Design review of the part built by this model. Coordinates are the model's own, in mm. A direction names the side the tool comes from. Round coordinates to 2 decimals unless told otherwise and drop trailing zeros. Order: outer loops, then holes, each group sorted by start corner. A loop starts at its lowest first (then second) coordinate and runs counter-clockwise, first axis right, second up.
from build123d import *

# Parameters (mm, degrees)
SKETCH1_W           = 50
SKETCH1_H           = 20
BOSS_EXTRUDE1_DEPTH = 40
SKETCH2_W           = 45
SKETCH2_H           = 75.2
CUT_EXTRUDE1_DEPTH  = 15
CUT_EXTRUDE2_REACH  = 86.41
SKETCH3_W           = 8
SKETCH3_H           = 3
SKETCH4_W           = 30
SKETCH4_H           = 60
CUT_EXTRUDE3_DEPTH  = 1


with BuildPart() as part:
    # Sketch1 → Boss-Extrude1 (new, symmetric)
    with BuildSketch(Plane.XY):
        Rectangle(SKETCH1_W, SKETCH1_H)
    extrude(amount=BOSS_EXTRUDE1_DEPTH, both=True)

    # Sketch2 → Cut-Extrude1 (cut)
    with BuildSketch(Plane(origin=(0, 10, 0), x_dir=(1, 0, 0), z_dir=(0, 1, 0))):
        with Locations((0, -1.4)):
            Rectangle(SKETCH2_W, SKETCH2_H)
    extrude(amount=-CUT_EXTRUDE1_DEPTH, mode=Mode.SUBTRACT)

    # Sketch3 → Cut-Extrude2 (cut, up to next)
    with BuildSketch(Plane.XY.offset(40), mode=Mode.PRIVATE) as cut_extrude2_sk1:
        with Locations((0, -3.5)):
            Rectangle(SKETCH3_W, SKETCH3_H)
    cut_extrude2_tool1 = extrude(cut_extrude2_sk1.sketch, amount=-CUT_EXTRUDE2_REACH, mode=Mode.PRIVATE) & part.part
    add(cut_extrude2_tool1.solids().sort_by_distance((0, -3.5, 40))[0], mode=Mode.SUBTRACT)

    # Sketch4 → Cut-Extrude3 (cut)
    with BuildSketch(Plane(origin=(0, -5, 0), x_dir=(1, 0, 0), z_dir=(0, 1, 0))):
        with Locations((0, -9)):
            Rectangle(SKETCH4_W, SKETCH4_H)
    extrude(amount=-CUT_EXTRUDE3_DEPTH, mode=Mode.SUBTRACT)


solid = part.part
1) Clearance check with a flat-ended pin moving along its axis: P1, Ø5, axis at x = -18.5, z = -7.5, coming from the +Y side. State where the tip first meets the part, or that it passes through.
Results:
P1: stops at y = -5
2) For faces 5 (the face through (-25, 0, 1)), 6 (the face through (0, 3, -36.2)), list the 3-axis set-ups (+Z, -Z, +X, -X, +Y, -Y) from which the entire face can be reached by the end or side of a thin tool; tool diameter is ignored.
Results:
face 5: +Z, -Z, -X, +Y, -Y
face 6: +Y
3) The part is to be moulded in two halves that separate along Z. For faces 1 (the face through (0, 0, -40)), 2 (the face through (0, -10, 1)), 3 (the face through (0, 0, 40)), 4 (the face through (0, 2, 39)), say which applies: released by +Z, released by -Z, zero draft, split by the parting line, or undercut.
Results:
face 1: released by -Z
face 2: zero draft
face 3: released by +Z
face 4: undercut
4) Take a section at C-C on x = -9. Give the boundary of the cut face in (y, z), plus the area to 3 significant figures.
Results:
outline: (-10, -40) - (10, -40) - (10, -36.2) - (-5, -36.2) - (-5, -21) - (-6, -21) - (-6, 39) - (10, 39) - (10, 40) - (-10, 40) - close
area: 412 mm2
5) To check wall thickness, follow line 1 along Z through (x, y) = (9, -0.5); line 2 along X through (y, z) = (7.5, 20); line 3 along Y through (x, z) = (-18.5, 2). State the ranges of each line that lie inside material, in increasing order.
Results:
line 1: z = -40 to -36.2, 39 to 40
line 2: x = -25 to -22.5, 22.5 to 25
line 3: y = -10 to -5
6) Take a section at D-D on z = -9.5. Give the boundary of the cut face in (x, y).
Results:
outline: (-25, -10) - (25, -10) - (25, 10) - (22.5, 10) - (22.5, -5) - (15, -5) - (15, -6) - (-15, -6) - (-15, -5) - (-22.5, -5) - (-22.5, 10) - (-25, 10) - close
7) Take a section at B-B on y = 1.5. Give the boundary of the cut face in (x, z).
Results:
outline: (-25, -40) - (25, -40) - (25, 40) - (-25, 40) - close; hole (-22.5, -36.2) - (22.5, -36.2) - (22.5, 39) - (-22.5, 39) - close
8) Take a section at A-A on x = 1.5. Give the boundary of the cut face in (y, z).
Results:
outline: (-10, -40) - (10, -40) - (10, -36.2) - (-5, -36.2) - (-5, -21) - (-6, -21) - (-6, 39) - (-5, 39) - (-5, 40) - (-10, 40) - close; (-2, 39) - (10, 39) - (10, 40) - (-2, 40) - close
